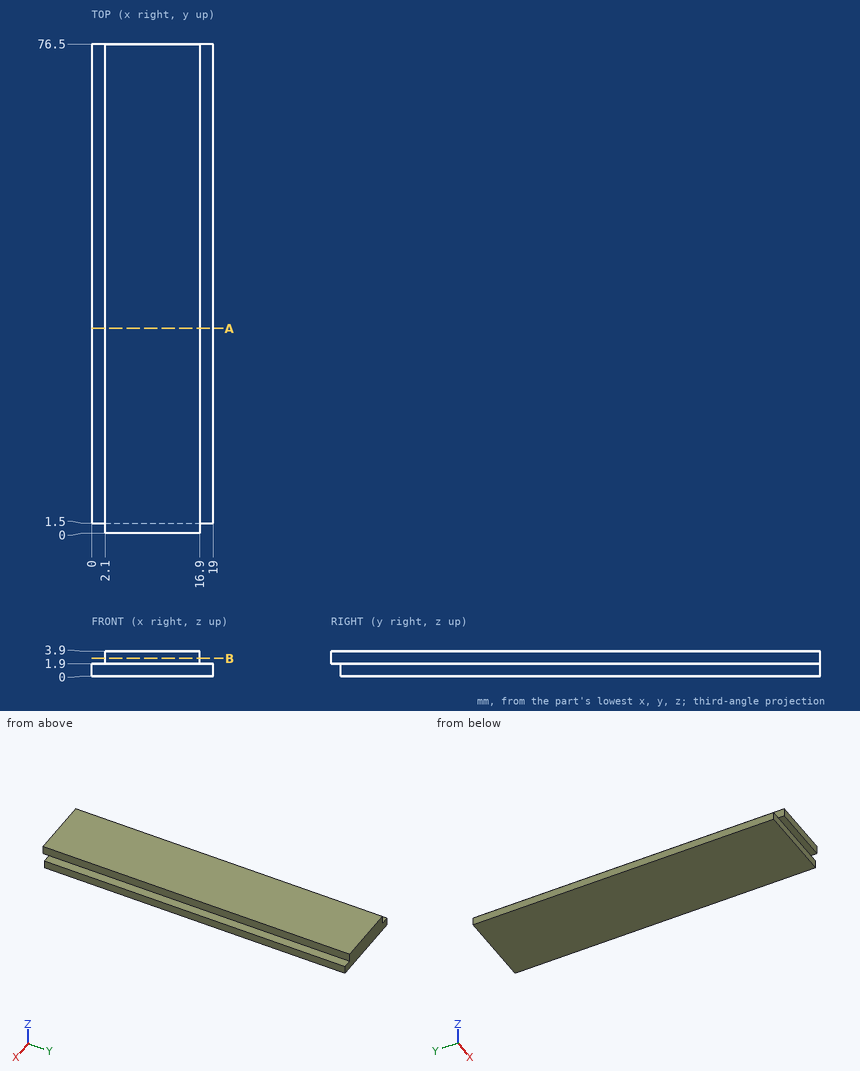
Job drawing, mm, ordinate dimensions from the low corner. One solid piece. Give positions to 0.01 mm unless a question says otherwise; leave off trailing zeros. Loops run counter-clockwise (first coordinate to the right, second up) from the corner with the lowest first, then second, coordinate; pieces in that order, holes last. Notation, with made-up numbers: (-34.5, 7.5) -> (24.5, 7.5) arc R31 cw to (24.5, 45.5) -> close; hole circle Ø7 at (12, 5). An arc over 180 degrees is marked (long way). Use a Markdown table: item, result. Add a question column.
(1) Wall check: line 1 along X through (y, z) = (30, 3.6); line 2 along Z through (x, y) = (2, 57); line 3 along Y through (x, z) = (12, 1.75). Give the ranges that are in metal, low to high.
(2) Slice it at B-B on z = 2.75. List the corners of the cut face in (x, y).
(3) Drop flat-ended pins along their axis: pin 1 Ø1.6 at (y, z) = (19.5, 3) entering from +X; pin 2 Ø1.5 at (x, z) = (11, 0.5) entering from -Y; pin 3 Ø1.1 at (x, y) = (1, 28.5) entering from +Z. Give the stop position or say it passes through.
(4) Slice it at A-A on y = 32. List the corners of the cut face in (x, z).
Filled sheet:
| question | item | result |
|---|---|---|
| 1 | line 1 | 2.1 to 16.9 |
| 1 | line 2 | 0 to 1.9 |
| 1 | line 3 | 1.5 to 76.5 |
| 2 | outline | (2.1, 0) -> (16.9, 0) -> (16.9, 76.5) -> (2.1, 76.5) -> close |
| 3 | pin 1 | x = 16.9 |
| 3 | pin 2 | y = 1.5 |
| 3 | pin 3 | z = 1.9 |
| 4 | outline | (0, 0) -> (19, 0) -> (19, 1.9) -> (16.9, 1.9) -> (16.9, 3.9) -> (2.1, 3.9) -> (2.1, 1.9) -> (0, 1.9) -> close |
